Autodesk Inventor part; units mm, degrees
ref_plane "YZ Plane" through (0, 0, 0) normal (1, 0, 0) x (0, 1, 0)
ref_plane "XZ Plane" through (0, 0, 0) normal (0, 1, 0) x (-1, 0, 0)
ref_plane "XY Plane" through (0, 0, 0) normal (0, 0, 1) x (1, 0, 0)
sketch "Boceto1" plane through (0, 0, 0) normal (0, 1, 0) x (-1, 0, 0)
  circle A0 centre (0.65, -0.45) radius 0.15
  line L0 (0.3, 0) -> (1.3, 0)
  line L1 (1.3, 0) -> (1.3, -1)
  line L2 (1.3, -1) -> (0.3, -1)
  line L3 (0.3, -1) -> (0, -1)
  line L4 (0, -1) -> (0, 0)
  line L5 (0, 0) -> (0.3, 0)
extrude "Extrusión1" add sketch "Boceto1" along normal blind 0.3
sketch "Boceto2" plane through (0, 0, 0) normal (0, -1, 0) x (1, 0, 0)
  line L0 (0, -1) -> (0, 0)
  line L1 (-0.3, -1) -> (0, -1)
  line L2 (0, 0) -> (-0.3, 0)
  line L3 (-0.3, 0) -> (-0.3, -1)
  line L4 (0, 0) -> (0, -1)
  line L5 (-0.3, -1) -> (0, -1)
  line L6 (0, -1) -> (0, 0)
  line L7 (0, 0) -> (-0.3, 0)
  line L8 (-0.3, 0) -> (-0.3, -1)
extrude "Extrusión2" add sketch "Boceto2" along normal blind 3.4
sketch "Boceto3" plane through (0, 0.3, 0) normal (1, 0, 0) x (0, 0, -1)
  line L0 (1, 0) -> (1, -3.7)
  line L1 (0, 0) -> (1, 0)
  line L2 (0, 0) -> (0, -3.7)
  line L3 (1, -3.7) -> (0, -3.7)
  line L4 (0, 0) -> (0, -3.7)
  line L5 (0, -3.7) -> (0, -3.4)
  line L6 (0, -3.4) -> (1, -3.4)
  line L7 (1, -3.4) -> (1, -3.7)
  line L8 (1, -3.7) -> (0, -3.7)
  line L9 (0, -3.7) -> (0, -3.4)
  point P0 (0, -0.3)
  dimension "d4" = 0.3
extrude "Extrusión3" add sketch "Boceto3" along normal blind 1.8 contours L0 L3 L2 L6
sketch "Boceto4" plane through (0, -3.4, 0) normal (0, -1, 0) x (1, 0, 0)
  line L0 (-0.3, 0) -> (1.8, 0)
  line L1 (-0.3, 0) -> (-0.3, -1)
  line L2 (-0.3, -1) -> (1.8, -1)
  line L3 (1.8, 0) -> (1.8, -1)
  circle A0 centre (0.5, -0.5) radius 0.15
  circle A1 centre (-6.552, -4.409) radius 0.15
  circle A2 centre (-5.952, -4.409) radius 0.15
  line L4 (0.5, -0.5) -> (1.1, -0.5)
  circle A3 centre (1.1, -0.5) radius 0.15
  point P0 (0, 0)
  dimension "d7" = 0.3
  dimension "d18" = 0.3
  dimension "d19" = 0.3
  dimension "d21" = 0.3
extrude "Extrusión4" cut sketch "Boceto4" against normal blind 1 contours A0 | A3
sketch "Boceto6" plane through (0, 0.3, 0) normal (0, 1, 0) x (1, 0, 0)
  line L0 (-1.3, 1) -> (-1.3, 0)
  line L1 (-1.3, 0.5) -> (-1.3, 3.4)
  line L2 (0, 3.4) -> (0, -2.4)
  line L3 (-1.3, -2.4) -> (-1.3, 0.5)
  circle A0 centre (-0.65, -2.4) radius 0.15
  circle A1 centre (-0.65, 3.4) radius 0.15
  line L4 (0, 3.4) -> (0, 4.1)
  line L5 (0, 4.1) -> (-1.3, 4.1)
  line L6 (-1.3, 4.1) -> (-1.3, 3.4)
  line L7 (-1.3, -2.4) -> (-1.3, -3.1)
  line L8 (-1.3, -3.1) -> (0, -3.1)
  line L9 (0, -3.1) -> (0, -2.4)
  point P0 (0, 0)
  dimension "d22" = 2.9
  dimension "d23" = 5.8
  dimension "d24" = 1.3
  dimension "d25" = 0.3
  dimension "d26" = 0.3
  dimension "d28" = 0.7
extrude "Extrusión5" add sketch "Boceto6" against normal blind 0.3
properties part number "soporteOdroid"
Work out the finished part from the listing and answer in its coordinate system (mm). A direction names the side the tool comes from. Give positions to 0.01 mm unless a question says otherwise; leave off trailing zeros. Loops run counter-clockwise (first coordinate to the right, second up) from the corner with the lowest first, then second, coordinate; pieces in that order, holes last. Notation, with made-up numbers: (21, 12.25) -> (71, 12.25) arc R16 cw to (71, 21.25) -> close; hole circle Ø7 at (32, -21). An arc over 180 degrees is marked (long way). One line per question, with ' | ' between items. Start each with the question number.
1) Section C-C, the plane x = 0.5 is taken. Determine the outline of the cut face in (y, z).
2) Straight lines are drawn through the part: L1, parallel to Z at x = -0.65, y = 0.1; L2, parallel to Z at x = 1.1, y = -3.25; L3, parallel to X at y = 0.1, z = -3.4. For each, find the intervals that lie inside material, in ascending order.
3) Section D-D, the plane z = -3.4 is taken. Determine the outline of the cut face in (x, y).
4) Section A-A, the plane x = -0.65 is taken. Determine the outline of the cut face in (y, z), then the cut area to 3 significant figures.
5) Section B-B, the plane z = -0.5 is taken. Determine the outline of the cut face in (x, y).
6) For faces 1 (the face through (-1, 0.3, -1)), 2 (the face through (-0.3, -1.7, -0.5)), 3 (the face through (0, -0.8, -0.5)), determine the directions among +Z, -Z, +X, -X, +Y, -Y from which every point of the face is accessible in a straight line to the end or side of a thin tool.
7) Each of these flat-tipped pins is pushed along its axis until it touches: pin 1 (1.1 mm diameter, centred on y = -2, z = -0.5, fed in from -X); pin 2 (1.1 mm diameter, centred on x = 1, z = -0.5, fed in from +Y); pin 3 (1 mm diameter, centred on x = -1, z = 1, fed in from -Y); pin 4 (1 mm diameter, centred on x = 1, y = -1, fed in from -Z). Where does it stop, or does it pass through?
Resolved:
1) outline: (-3.4, -1) -> (-3.1, -1) -> (-3.1, -0.65) -> (-3.4, -0.65) -> close; (-3.4, -0.35) -> (-3.1, -0.35) -> (-3.1, 0) -> (-3.4, 0) -> close
2) L1: -4.1 to -3.55, -3.25 to 2.25, 2.55 to 3.1 | L2: -1 to -0.65, -0.35 to 0 | L3: -1.3 to -0.8, -0.5 to 0
3) outline: (-1.3, 0) -> (-0.8, 0) -> (-0.8, 0.3) -> (-1.3, 0.3) -> close; (-0.5, 0) -> (0, 0) -> (0, 0.3) -> (-0.5, 0.3) -> close
4) outline: (0, -4.1) -> (0.3, -4.1) -> (0.3, -3.55) -> (0, -3.55) -> close; (0, -3.25) -> (0.3, -3.25) -> (0.3, 2.25) -> (0, 2.25) -> close; (0, 2.55) -> (0.3, 2.55) -> (0.3, 3.1) -> (0, 3.1) -> close | area: 1.98 mm2
5) outline: (-1.3, 0) -> (-0.3, 0) -> (-0.3, -3.4) -> (0.35, -3.4) -> (0.35, -3.1) -> (0, -3.1) -> (0, 0.3) -> (-1.3, 0.3) -> close; (0.65, -3.4) -> (0.95, -3.4) -> (0.95, -3.1) -> (0.65, -3.1) -> close; (1.25, -3.4) -> (1.8, -3.4) -> (1.8, -3.1) -> (1.25, -3.1) -> close
6) face 1: +Z, -Z, +X, -X, +Y | face 2: +Z, -Z, -X, -Y | face 3: +Z, -Z, +X, +Y
7) pin 1: x = -0.3 | pin 2: y = -3.1 | pin 3: y = 0 | pin 4: through
